The model under review builds one solid part; all positions refer to its coordinate system, in mm. A direction names the side the tool comes from. Round coordinates to 2 decimals unless told otherwise and drop trailing zeros. Loops run counter-clockwise (first coordinate to the right, second up) from the corner with the lowest first, then second, coordinate; pieces in that order, holes last. Notation, with made-up numbers: M 45.5,-40 L 74.5,-40 A21 ccw 74.5,-30 Z; hole C 88.25,52 d4. An arc over 180 degrees is marked long. Answer in a Markdown table with one row per item. Add a question column.
from build123d import *

# Parameters (mm, degrees)
SKETCH1_R           = 1.5
BOSS_EXTRUDE1_DEPTH = 4
CUT_EXTRUDE2_DEPTH  = 26.059928172
CIRPATTERN1_COUNT   = 12
SKETCH3_W           = 9.640063732
SKETCH3_H           = 5
BOSS_EXTRUDE6_DEPTH = 4
SKETCH4_R           = 2.5
CUT_EXTRUDE3_DEPTH  = 26.059928172


with BuildPart() as part:
    # Sketch1 → Boss-Extrude1 (new body)
    with BuildSketch(Plane.XY):
        with BuildLine():
            Line((-18, 2.5), (12.545643943, 2.5))
            ThreePointArc((12.545643943, 2.5), (24, 0), (12.545643943, -2.5))
            Line((12.545643943, -2.5), (-18, -2.5))
            ThreePointArc((-18, -2.5), (-20.5, 0), (-18, 2.5))
        make_face()
        with Locations((-18, 0)):
            Circle(SKETCH1_R, mode=Mode.SUBTRACT)
    extrude(amount=BOSS_EXTRUDE1_DEPTH)

    # Sketch2 → Cut-Extrude2 (cut, through all)
    with BuildSketch(Plane.XY.offset(4)):
        with BuildLine():
            Line((18.72, 5.06), (18.654523502, 4.81))
            ThreePointArc((18.654523502, 4.81), (19.09327028, 4.062778187), (19.840492093, 4.501524965))
            Line((19.840492093, 4.501524965), (19.906461709, 4.742088543))
            ThreePointArc((19.906461709, 4.742088543), (20.342216866, 5.236479445), (21, 5.196152423))
            ThreePointArc((21, 5.196152423), (19.568400179, 5.853349156), (18, 6))
            ThreePointArc((18, 6), (18.589879661, 5.706078038), (18.72, 5.06))
        make_face()
    cut_extrude2 = extrude(amount=-CUT_EXTRUDE2_DEPTH, mode=Mode.SUBTRACT)

    # CirPattern1: Cut-Extrude2 ×12 about axis
    cirpattern1_axis = Axis((18, 0, 0), (0, 0, 1))
    for i in range(1, CIRPATTERN1_COUNT):
        add(cut_extrude2.rotate(cirpattern1_axis, i * 360 / CIRPATTERN1_COUNT), mode=Mode.SUBTRACT)

    # Sketch3 → Boss-Extrude6 (add)
    with BuildSketch(Plane.XY.offset(4)):
        with Locations((15.25827781, 0)):
            Rectangle(SKETCH3_W, SKETCH3_H)
    extrude(amount=-BOSS_EXTRUDE6_DEPTH)

    # Sketch4 → Cut-Extrude3 (cut, through all)
    with BuildSketch(Plane.XY.offset(4)):
        with Locations((18, 0)):
            Circle(SKETCH4_R)
    extrude(amount=-CUT_EXTRUDE3_DEPTH, mode=Mode.SUBTRACT)


solid = part.part
1. Machinability: for faces 1 (the flat face through (-2, -2.5, 2)), 2 (the cylindrical face through (-19.5, 0.07, 1.97)), which of the approach directions +Z, -Z, +X, -X, +Y, -Y give a long, thin tool a straight path to every point of the face, cutting with its end or side? Answer none if there is none.
2. Mouldability with a two-part tool opening along Y and no side actions: class faces 3 (the flat face through (4, 0, 4)), 4 (the cylindrical face through (22.06, 1.1, 2.03)), 5 (the cylindrical face through (23.24, 2.35, 2.03)), 6 (the cylindrical face through (22.656, -3.363, 2.028)) as released by +Y, released by -Y, zero draft, split by the parting line, or undercut.
3. To check wall thickness, follow probe 1 along X at (y, z) = (4.5, 1); probe 2 along X at (y, z) = (-3, 2.45); probe 3 along Y at (x, z) = (18, 3.8). State the ranges of each line that lie inside material, in increasing order.
4. For pin 1 Ø6 at (x, y) = (18, 0) entering from +Z; pin 2 Ø2 at (y, z) = (-4, 3) entering from -X; pin 3 Ø1.2 at (x, z) = (-8.5, 2) entering from +Y, all flat-tipped, find the tip position at first contact; note any pin that passes through.
5. Take a section at A-A, the plane z = 1.2. State how many separate pieces and enclosed holes the cut face has, and give its area (3 significant figures).
6. Take a section at B-B, the plane x = -1. State the section outline as (y, z) points.
Check sheet entries:
| question | item | result |
|---|---|---|
| 1 | face 1 | +Z, -Z, -X, -Y |
| 1 | face 2 | +Z, -Z |
| 2 | face 3 | zero draft |
| 2 | face 4 | undercut |
| 2 | face 5 | undercut |
| 2 | face 6 | released by -Y |
| 3 | probe 1 | x = 14.63 to 16.16, 17.35 to 18.65, 19.84 to 21.37 |
| 3 | probe 2 | x = 12.8 to 14.13, 15.05 to 20.95, 21.87 to 23.2 |
| 3 | probe 3 | y = -6 to -2.5, 2.5 to 6 |
| 4 | pin 1 | stops at z = 4 |
| 4 | pin 2 | stops at x = 12.8 |
| 4 | pin 3 | stops at y = 2.5 |
| 5 | separate pieces | 1 |
| 5 | enclosed holes | 2 |
| 5 | area | 223 mm^2 |
| 6 | outline | M -2.5,0 L 2.5,0 L 2.5,4 L -2.5,4 Z |
